Input: part model. Units: mm. Frame: model coordinates. Round coordinates to 2 decimals unless told otherwise and drop trailing zeros. Loops run counter-clockwise (first coordinate to the right, second up) from the corner with the lowest first, then second, coordinate; pieces in that order, holes last. Notation, with made-up numbers: M -2.5,-13.5 L 40.5,-13.5 A19 ccw 40.5,21.5 Z; hole C 83,-5 d10. An arc over 180 degrees is marked long. Put each result on its own line as item: value. Start each with the question number.
1) Section C-C on y = 4.1. Output: boundary loops of the cut face in (x, z).
2) Section B-B on x = -7. Output: boundary loops of the cut face in (y, z).
3) Line query: probe 1 along Z at (x, y) = (-38.5, 1.1); probe 2 along X at (y, z) = (2.1, 4); probe 3 along Z at (x, y) = (-7, 3.7). Output: solid intervals per line, ascending.
4) Pin query (flat end, axial travel): pin 1 (1.5 mm diameter, centred on y = 4, z = -52, fed in from -X); pin 2 (1.5 mm diameter, centred on x = 38, y = 3, fed in from +Z); pin 3 (1.5 mm diameter, centred on x = 38, y = 4, fed in from -Z). Return the tip coordinate at first contact, or that it passes through.
5) Section A-A on z = 9. Output: boundary loops of the cut face in (x, y), plus the area to 3 significant figures.
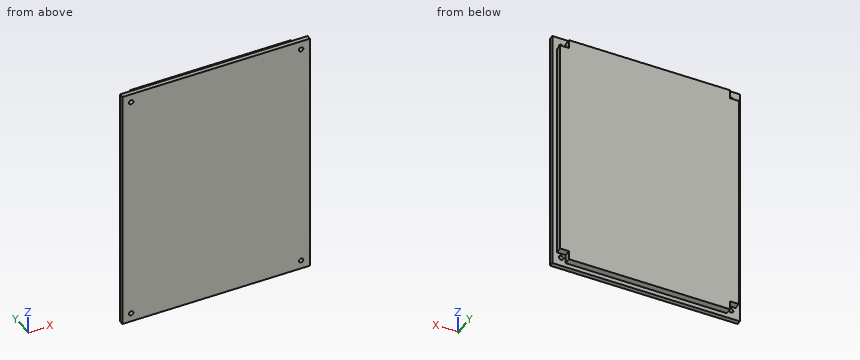
Autodesk Inventor part; units mm, degrees
ref_plane "YZ Plane" through (0, 0, 0) normal (1, 0, 0) x (0, 1, 0)
ref_plane "XY Plane" through (0, 0, 0) normal (0, 0, 1) x (1, 0, 0)
sketch "Sketch7" plane through (0, 0, 0) normal (0, 1, 0) x (-1, 0, 0)
  line L0 (-42.5, 57) -> (42.5, 57)
  line L1 (42.5, 57) -> (42.5, -57)
  line L2 (42.5, -57) -> (-42.5, -57)
  line L3 (-42.5, -57) -> (-42.5, 57)
  line L4 (-42.5, 57) -> (42.5, -57) construction
  line L5 (42.5, 57) -> (-42.5, -57) construction
  line L6 (-40.5, 55) -> (40.5, -55) construction
  line L7 (40.5, 55) -> (-40.5, -55) construction
  line L8 (36.5, 55) -> (36.5, 51)
  line L9 (36.5, 51) -> (40.5, 51)
  line L10 (36.5, -55) -> (36.5, -51)
  line L11 (36.5, -51) -> (40.5, -51)
  line L12 (-36.5, -55) -> (-36.5, -51)
  line L13 (-36.5, -51) -> (-40.5, -51)
  line L14 (-36.5, 55) -> (-36.5, 51)
  line L15 (-36.5, 51) -> (-40.5, 51)
  line L16 (40.5, -51) -> (40.5, 51)
  line L17 (36.5, 55) -> (-36.5, 55)
  line L18 (-40.5, 51) -> (-40.5, -51)
  line L19 (-36.5, -55) -> (36.5, -55)
  circle A0 centre (38.5, 53) radius 1
  circle A1 centre (38.5, -53) radius 1
  circle A2 centre (-38.5, 53) radius 1
  circle A3 centre (-38.5, -53) radius 1
  point P0 (0, 0)
  dimension "d36" = 85
  dimension "d37" = 114
  dimension "d38" = 81
  dimension "d39" = 110
  dimension "d40" = 4
  dimension "d41" = 4
  dimension "d42" = 4
  dimension "d43" = 4
  dimension "d44" = 4
  dimension "d45" = 4
  dimension "d46" = 4
  dimension "d47" = 4
  dimension "d48" = 2
  dimension "d49" = 2
  dimension "d50" = 2
  dimension "d51" = 2
extrude "Extrusion4" add sketch "Sketch7" along normal blind 2
sketch "Sketch8" plane through (0, 0, 0) normal (0, 1, 0) x (-1, 0, 0)
  point P0 (0, 0)
sketch "Sketch9" plane through (0, 0, 0) normal (0, 1, 0) x (-1, 0, 0)
  line L0 (36.5, 55) -> (36.5, 51)
  line L1 (36.5, 51) -> (40.5, 51)
  line L2 (36.5, 51) -> (40.5, 51)
  line L3 (40.5, -51) -> (36.5, -51)
  line L4 (40.5, 51) -> (40.5, -51)
  line L5 (40.5, -51) -> (36.5, -51)
  line L6 (36.5, -51) -> (36.5, -55)
  line L7 (36.5, -51) -> (36.5, -55)
  line L8 (36.5, -55) -> (-36.5, -55)
  line L9 (36.5, -55) -> (-36.5, -55)
  line L10 (-36.5, -55) -> (-36.5, -51)
  line L11 (-40.5, -51) -> (-40.5, 51)
  line L12 (-36.5, -51) -> (-40.5, -51)
  line L13 (-40.5, -51) -> (-40.5, 51)
  line L14 (-40.5, 51) -> (-36.5, 51)
  line L15 (-40.5, 51) -> (-36.5, 51)
  line L16 (-36.5, 55) -> (36.5, 55)
  line L17 (-36.5, 51) -> (-36.5, 55)
  line L18 (-36.5, 55) -> (36.5, 55)
  line L19 (36.5, 55) -> (36.5, 51)
  point P0 (0, 0)
extrude "Extrusion5" add sketch "Sketch9" along normal blind 5
properties part number "bottom plant watner"
Geometry results:
1. outline: M -40.5,-51 L -36.5,-51 L -36.5,-55 L 36.5,-55 L 36.5,-51 L 40.5,-51 L 40.5,51 L 36.5,51 L 36.5,55 L -36.5,55 L -36.5,51 L -40.5,51 Z
2. outline: M 0,-57 L 2,-57 L 2,-55 L 5,-55 L 5,55 L 2,55 L 2,57 L 0,57 Z
3. probe 1: z = -57 to -54, -52 to 52, 54 to 57
3. probe 2: x = -40.5 to 40.5
3. probe 3: z = -55 to 55
4. pin 1: stops at x = -36.5
4. pin 2: stops at z = 51
4. pin 3: stops at z = -51
5. outline: M -42.5,0 L 42.5,0 L 42.5,2 L 40.5,2 L 40.5,5 L -40.5,5 L -40.5,2 L -42.5,2 Z
5. area: 413 mm²
